The listing builds one solid part. Answer for the finished solid, in the listing's coordinates (mm). Face numbers are marked on the shaded views. A direction names the side the tool comes from. Round coordinates to 2 decimals unless told otherwise and drop trailing zeros. Order: outer loops, then holes, each group sorted by start corner. A loop starts at its lowest first (then second) coordinate and runs counter-clockwise, first axis right, second up. Notation, with made-up numbers: M 76.5,-35.75 L 95.5,-35.75 A16 cw 95.5,-13.75 Z; hole C 53.25,54 d8. An arc over 180 degrees is marked long. Put each result on its own line as item: value. Start each with the question number.
1. The part is cut by section B-B (x = 38.1). Give the vertices of the cut face in (y, z) (3 decimals).
2. The part is cut by section D-D (y = -17.5). Give the vertices of the cut face in (x, z).
3. The part is cut by section C-C (z = 60.5). Give the vertices of the cut face in (x, y), then the cut area to 3 significant figures.
4. Consider line 1 (X direction, y = -13, z = 20.5); line 2 (Y direction, x = 15, z = 17.5); line 3 (X direction, y = -33, z = 94) (3 decimals). Determine where each line is inside the solid, lowest interval first.
5. The part is cut by section A-A (z = 23.5). Count the separate pieces of the cut face and the enclosed holes in it, then the cut area to 3 significant figures.
6. Each of these flat-tipped pins is pushed along its axis until it touches: pin 1 Ø15 at (y, z) = (-44.5, 61.5) entering from +X; pin 2 Ø10 at (x, y) = (35, -42.5) entering from +Z; pin 3 Ø18.5 at (x, y) = (15.875, -85.725) entering from +Z. Where does it stop, or does it pass through?
7. Which of the six approach directions +Z, -Z, +X, -X, +Y, -Y give full straight-line access (tool end or side, diameter ignored) to the marked faces 1, 2, 3, 4 and 5?
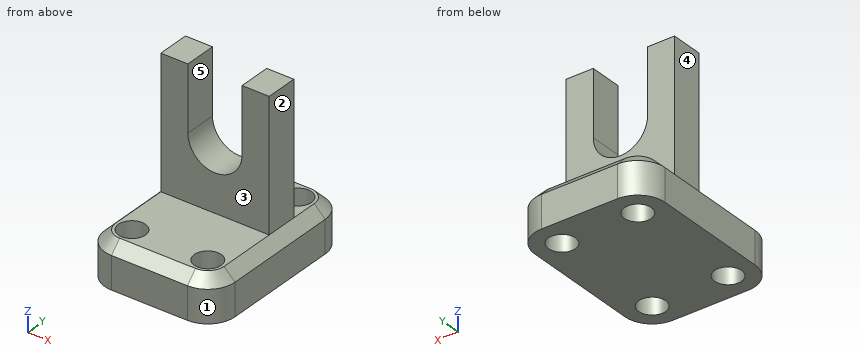
from build123d import *

# Parameters (mm, degrees)
F1_DEPTH = 25.4
F2_D     = 15.875
F3_SIZE  = 6.35
F4_W     = 63.5
F4_H     = 19.05
F5_DEPTH = 76.2
F7_DEPTH = 25.4


with BuildPart() as f1:
    # F0 (on Top) → F1 (new body)
    with BuildSketch(Plane.XY):
        with BuildLine():
            Line((60.325, 0), (15.875, 0))
            ThreePointArc((15.875, 0), (4.6496798487, -4.6496798487), (0, -15.875))
            Line((0, -15.875), (0, -85.725))
            ThreePointArc((0, -85.725), (4.6496798487, -96.9503201513), (15.875, -101.6))
            Line((15.875, -101.6), (60.325, -101.6))
            ThreePointArc((60.325, -101.6), (71.5503201513, -96.9503201513), (76.2, -85.725))
            Line((76.2, -85.725), (76.2, -15.875))
            ThreePointArc((76.2, -15.875), (71.5503201513, -4.6496798487), (60.325, 0))
        make_face()
    extrude(amount=F1_DEPTH)

    # F2 (through all)
    with Locations(Plane(origin=(0, 0, 0), x_dir=(1, 0, 0), z_dir=(0, 0, -1))):
        with Locations((15.875, 15.875), (60.325, 15.875), (60.325, 85.725), (15.875, 85.725)):
            Hole(F2_D / 2)

    # F3
    f3_edges = [f1.edges().sort_by_distance(p)[0] for p in [
        (4.64968, -4.64968, 25.4),
    ]]
    chamfer(f3_edges, length=F3_SIZE)

    # F4 (on face) → F5 (join)
    with BuildSketch(Plane.XY.offset(25.4)):
        with Locations((38.1, -41.275)):
            Rectangle(F4_W, F4_H)
    extrude(amount=F5_DEPTH)

    # F6 (on face) → F7 (cut)
    with BuildSketch(Plane.XZ.offset(50.8)):
        with BuildLine():
            Line((53.975, 63.5), (53.975, 101.6))
            Line((53.975, 101.6), (22.225, 101.6))
            Line((22.225, 101.6), (22.225, 63.5))
            ThreePointArc((22.225, 63.5), (38.1, 79.375), (53.975, 63.5))
        make_face()
        with BuildLine():
            ThreePointArc((22.225, 63.5), (38.1, 47.625), (53.975, 63.5))
            ThreePointArc((53.975, 63.5), (38.1, 79.375), (22.225, 63.5))
        make_face()
    extrude(amount=-F7_DEPTH, mode=Mode.SUBTRACT)


solid = f1.part
Resolved:
1. outline: M -101.6,0 L 0,0 L 0,19.05 L -6.35,25.4 L -31.75,25.4 L -31.75,47.625 L -50.8,47.625 L -50.8,25.4 L -95.25,25.4 L -101.6,19.05 Z
2. outline: M 0,0 L 8.11,0 L 8.11,25.4 L 6.35,25.4 L 0,19.05 Z; M 23.64,0 L 52.56,0 L 52.56,25.4 L 23.64,25.4 Z; M 68.09,0 L 76.2,0 L 76.2,19.05 L 69.85,25.4 L 68.09,25.4 Z
3. outline: M 6.35,-50.8 L 22.51,-50.8 L 22.51,-31.75 L 6.35,-31.75 Z; M 53.69,-50.8 L 69.85,-50.8 L 69.85,-31.75 L 53.69,-31.75 Z
3. area: 616 mm2
4. line 1: 1.74 to 8.48, 23.27 to 52.93, 67.72 to 74.46
4. line 2: -101.58 to -93.61, -77.84 to -23.76, -7.99 to -0.02
4. line 3: 6.35 to 22.225, 53.975 to 69.85
5. separate pieces: 1
5. enclosed holes: 4
5. area: 5,330 mm2
6. pin 1: x = 69.85
6. pin 2: z = 49.85
6. pin 3: z = 25.4
7. face 1: +Z, -Z, +X, -Y
7. face 2: +Z, +X, +Y, -Y
7. face 3: +Z, +X, -X, -Y
7. face 4: +Z, -X, +Y, -Y
7. face 5: +Z, +Y, -Y
